Check sheet for the modelled part. Datum: model origin and axes. Units: mm. A direction names the side the tool comes from. Coordinates: 2 decimals unless noted, no trailing zeros. Loops run counter-clockwise (first coordinate to the right, second up) from the corner with the lowest first, then second, coordinate; pieces in that order, holes last. Notation, with made-up numbers: M 40.25,73 L 66.25,73 A26 cw 66.25,93 Z; hole C 24.5,-23.5 d1. An arc over 180 degrees is marked long. Use CSV: the item, a comma, the result in double quotes. Start each with the question number.
(1) Set-up check for faces 4 (the flat face through (38.1, 0, 77)), 5 (the flat face through (1, -25.4, 28)), 6 (the flat face through (-57, 6.35, 95)): record each of +Z, -Z, +X, -X, +Y, -Y from which the full face is reachable in a straight line by a thin tool's end or side.
(2) Draft check along Z on faces 1 (the flat face through (57, 0, 88.9)), 2 (the flat face through (76.2, 0, 66)), 3 (the cylindrical face through (-70.47, -0.36, 5.43)). Enter one of: pulls with the +Z half, pulls with the -Z half, needs draft (parallel to the pull), parting line crosses it, or undercut.
(3) Section check B-B on z = 95. Record the cut outline in (x, y), and give its area (3 significant figures).
(4) Go/stop test with flat-tipped pins: pin 1 Ø15 at (x, y) = (18.5, 1) entering from +Z; pin 2 Ø4 at (x, y) = (66, 2) entering from -Z; pin 3 Ø1 at (x, y) = (57.5, -17) entering from +Z. Record where each tip stops, or that it passes through.
(5) Section check C-C on x = -42. Record the cut outline in (y, z).
(6) Section check D-D on y = -16.5. Record the cut outline in (x, z), and give its area (3 significant figures).
(7) Scan lines: line 1 (X direction, y = -20, z = 52); line 2 (Z direction, x = -7, y = -13); line 3 (Z direction, x = 39, y = 2). Record each from-to range of solid material in increasing order.
(8) Section check A-A on z = 61. Record the cut outline in (x, y), and give its area (3 significant figures).
from build123d import *

# Parameters (mm, degrees)
F1_DEPTH = 25.4
F3_W     = 12.7
F3_H     = 12.7
F4_DEPTH = 152.401


with BuildPart() as f1:
    # F0 (on Front) → F1 (new body, symmetric)
    with BuildSketch(Plane.XZ):
        with BuildLine():
            Line((0, 38.1), (0, 0))
            Line((0, 0), (38.1, 0))
            Line((38.1, 0), (57.15, 0))
            ThreePointArc((57.15, 0), (70.620384, 5.579616), (76.2, 19.05))
            Line((76.2, 19.05), (76.2, 38.1))
            Line((76.2, 38.1), (76.2, 114.3))
            Line((76.2, 114.3), (38.1, 114.3))
            Line((38.1, 114.3), (38.1, 38.1))
            Line((38.1, 38.1), (0, 38.1))
        make_face()
    extrude(amount=F1_DEPTH, both=True)

    # F2: F1 across plane


with BuildPart() as f1_1:
    add(f1.part)
    add(f1.part.mirror(Plane.YZ))

    # F3 (on face) → F4 (cut, through all)
    with BuildSketch(Plane(origin=(-76.2, 0, 0), x_dir=(0, -1, 0), z_dir=(-1, 0, 0))):
        with BuildLine():
            ThreePointArc((-25.4, 97.999742), (-15.090215, 109.874442), (0, 114.3))
            Line((0, 114.3), (-25.4, 114.3))
            Line((-25.4, 114.3), (-25.4, 97.999742))
        make_face()
        with BuildLine():
            ThreePointArc((0, 114.3), (15.090215, 109.874442), (25.4, 97.999742))
            Line((25.4, 97.999742), (25.4, 114.3))
            Line((25.4, 114.3), (0, 114.3))
        make_face()
        with Locations((0, 95.25)):
            Rectangle(F3_W, F3_H)
    extrude(amount=-F4_DEPTH, mode=Mode.SUBTRACT)


solid = f1_1.part
Outcome:
1,face 4,"+Z, +Y, -Y"
1,face 5,"+Z, -Z, +X, -X, -Y"
1,face 6,"+X, -X"
2,face 1,"undercut"
2,face 2,"needs draft"
2,face 3,"pulls with the -Z half"
3,outline,"M -76.2,-25.4 L -38.1,-25.4 L -38.1,-6.35 L -76.2,-6.35 Z; M -76.2,6.35 L -38.1,6.35 L -38.1,25.4 L -76.2,25.4 Z; M 38.1,-25.4 L 76.2,-25.4 L 76.2,-6.35 L 38.1,-6.35 Z; M 38.1,6.35 L 76.2,6.35 L 76.2,25.4 L 38.1,25.4 Z"
3,area,"2,900 mm²"
4,pin 1,"stops at z = 38.1"
4,pin 2,"stops at z = 1.27"
4,pin 3,"stops at z = 108.91"
5,outline,"M -25.4,0 L 25.4,0 L 25.4,98 A27.94 ccw 0,114.3 A27.94 ccw -25.4,98 Z; hole M -6.35,88.9 L 6.35,88.9 L 6.35,101.6 L -6.35,101.6 Z"
6,outline,"M -76.2,19.05 A19.05 ccw -57.15,0 L 57.15,0 A19.05 ccw 76.2,19.05 L 76.2,108.91 L 38.1,108.91 L 38.1,38.1 L -38.1,38.1 L -38.1,108.91 L -76.2,108.91 Z"
6,area,"11,000 mm²"
7,line 1,"x = -76.2 to -38.1, 38.1 to 76.2"
7,line 2,"z = 0 to 38.1"
7,line 3,"z = 0 to 88.9, 101.6 to 114.23"
8,outline,"M -76.2,-25.4 L -38.1,-25.4 L -38.1,25.4 L -76.2,25.4 Z; M 38.1,-25.4 L 76.2,-25.4 L 76.2,25.4 L 38.1,25.4 Z"
8,area,"3,870 mm²"
